```python
from build123d import *

# Parameters (mm, degrees)
SKETCH1_W = 13.208
SKETCH1_H = 15.875


with BuildPart() as part:
    # Sketch1 → Revolve1 (revolve)
    with BuildSketch(Plane(origin=(0, 0, 0), x_dir=(1, 0, 0), z_dir=(0, 1, 0)), mode=Mode.PRIVATE) as revolve1_sk:
        with BuildLine():
            Line((-281.178, 12.7), (-281.178, 0))
            Line((-281.178, 0), (281.178, 0))
            Line((281.178, 0), (281.178, 26.9875))
            Line((281.178, 26.9875), (-278.003, 26.9875))
            ThreePointArc((-278.003, 26.9875), (-280.24806403, 26.05756403), (-281.178, 23.8125))
            Line((-281.178, 23.8125), (-281.178, 12.7))
        make_face()
        with BuildLine():
            Line((-296.418, 11.1125), (-296.418, 0))
            Line((-296.418, 0), (-281.178, 0))
            Line((-281.178, 0), (-281.178, 12.7))
            Line((-281.178, 12.7), (-294.8305, 12.7))
            ThreePointArc((-294.8305, 12.7), (-295.953032015, 12.235032015), (-296.418, 11.1125))
        make_face()
        Polygon((281.178, 26.9875), (281.178, 0), (290.703, 0), (290.703, 15.875), (290.703, 28.8925), (281.178, 28.8925), align=None)
        with Locations((297.307, 7.9375)):
            Rectangle(SKETCH1_W, SKETCH1_H)
    revolve(revolve1_sk.sketch.rotate(Axis((-319.562207996, 0, 0), (1, 0, 0)), 180), axis=Axis((-319.562207996, 0, 0), (1, 0, 0)))


solid = part.part
```
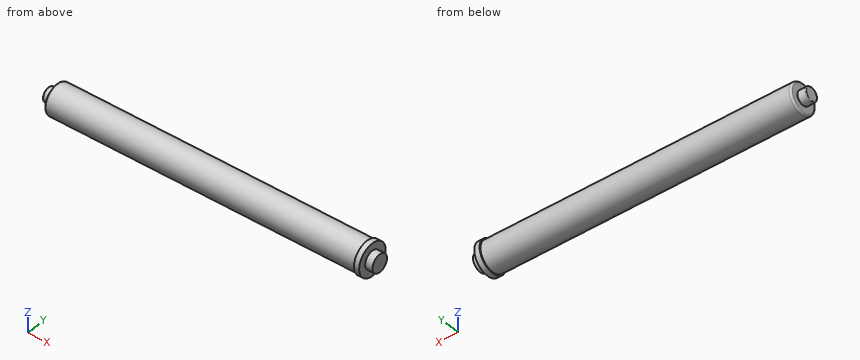
Model file for the job. Use its own axes, mm. Round coordinates to 2 decimals unless told otherwise and drop trailing zeros. Order: outer loops, then holes, each group sorted by start corner. A loop starts at its lowest first (then second) coordinate and runs counter-clockwise, first axis right, second up. Notation, with made-up numbers: M 26,56 L 65,56 A33 ccw 65,85 Z; hole C -28.5,25 d9. An arc over 180 degrees is marked long. Use CSV: the item, a comma, the result in double quotes.
Item 1: Pin check, flat tips, straight feed: pin 1 (4 mm diameter, centred on x = 230.5, y = -17.5, fed in from +Z); pin 2 (2 mm diameter, centred on x = 54.5, z = 13.5, fed in from +Y); pin 3 (1 mm diameter, centred on x = -141, y = -19, fed in from -Z); pin 4 (17.5 mm diameter, centred on y = -10, z = -14, fed in from +X). Stop position of each tip, or through.
Worked answers:
pin 1,"z = 22.09"
pin 2,"y = 23.92"
pin 3,"z = -19.65"
pin 4,"x = 303.91"
Item 2: Probe probe 1 along Y at (x, z) = (-62.5, 1.5); probe 2 along X at (y, z) = (-5.5, 19); probe 3 along Y at (x, z) = (37.5, 1). List the from-to ranges inside material, lowest first.
Worked answers:
probe 1,"-26.95 to 26.95"
probe 2,"-281.18 to 290.7"
probe 3,"-26.97 to 26.97"
Item 3: Saw through at C-C (x = -240). List the corners of the cut face in (y, z) (1 decimal), plus the area to 3 significant figures.
Worked answers:
outline,"C 0,0 d54"
area,"2,290 mm²"
